from build123d import *

# Parameters (mm, degrees)
SKETCH1_R           = 5.5
BOSS_EXTRUDE1_DEPTH = 11
SKETCH3_R           = 15
BOSS_EXTRUDE2_DEPTH = 2
SKETCH4_R           = 15.011076053
SKETCH4_R_2         = 13.011076053
BOSS_EXTRUDE3_DEPTH = 59
SKETCH5_R           = 15.011076053
BOSS_EXTRUDE4_DEPTH = 2
CAVITY1_OUTLINE_R   = 1.25
CAVITY1_DEPTH       = 8
SKETCH6_R           = 1.25
CUT_EXTRUDE1_DEPTH  = 8


# Read off the part's stored shape, not the designer's step: Cavity1
with BuildPart() as part:
    # Sketch1 → Boss-Extrude1 (new body)
    with BuildSketch(Plane.XY):
        with Locations((0.700759494, -0.350379747)):
            Circle(SKETCH1_R)
    boss_extrude1 = extrude(amount=BOSS_EXTRUDE1_DEPTH)

    # Sketch3 → Boss-Extrude2 (add)
    with BuildSketch(Plane.XY.offset(11)):
        with Locations((0.700759494, -0.350379747)):
            Circle(SKETCH3_R)
    extrude(amount=BOSS_EXTRUDE2_DEPTH)

    # Sketch4 → Boss-Extrude3 (add)
    with BuildSketch(Plane.XY.offset(13)):
        with Locations((0.700759494, -0.350379747)):
            Circle(SKETCH4_R)
        with Locations((0.700759494, -0.350379747)):
            Circle(SKETCH4_R_2, mode=Mode.SUBTRACT)
    extrude(amount=BOSS_EXTRUDE3_DEPTH)

    # Sketch5 → Boss-Extrude4 (add)
    with BuildSketch(Plane.XY.offset(72)):
        with Locations((0.700759494, -0.350379747)):
            Circle(SKETCH5_R)
    extrude(amount=BOSS_EXTRUDE4_DEPTH)

    # Mirror1: Boss-Extrude1 across plane
    add(boss_extrude1.mirror(Plane.XY.offset(42.5)))

    # Cavity1 outline → Cavity1 (cut)
    with BuildSketch(Plane.XY):
        with BuildLine():
            Line((3.338761962, -0.602258645), (0.613426942, 2.29818081))
            ThreePointArc((0.613426942, 2.29818081), (-1.113870906, 1.580841761), (-1.937242974, -0.098500849))
            Line((-1.937242974, -0.098500849), (0.788092045, -2.998940304))
            ThreePointArc((0.788092045, -2.998940304), (2.515389893, -2.281601255), (3.338761962, -0.602258645))
        make_face()
        with Locations((0.700759494, -0.350379747)):
            Circle(CAVITY1_OUTLINE_R, mode=Mode.SUBTRACT)
    extrude(amount=CAVITY1_DEPTH, mode=Mode.SUBTRACT)

    # Sketch6 → Cut-Extrude1 (cut)
    with BuildSketch(Plane(origin=(0, 0, 0), x_dir=(-1, 0, 0), z_dir=(0, 0, -1))):
        with Locations((-0.700759494, -0.350379747)):
            Circle(SKETCH6_R)
    extrude(amount=-CUT_EXTRUDE1_DEPTH, mode=Mode.SUBTRACT)


solid = part.part
Design review of the part built by this model. Coordinates are the model's own, in mm. A direction names the side the tool comes from. Round coordinates to 2 decimals unless told otherwise and drop trailing zeros. Write each loop counter-clockwise with the first axis right and the second up, starting at its lowest first coordinate (ties: lowest second). Pieces come first, ordered by that corner, then holes.
Item 1: Consider section C-C on z = 6.5. Give the boundary of the cut face in (x, y), and give its area (3 significant figures).
Item 2: Draft analysis for pull direction Z (two halves, no side actions). For faces 5 (the flat face through (1, 0, 8)), 6 (the flat face through (1, 0, 13)), 7 (the cylindrical face through (-0.49, -5.72, 79.58)), state which applies: released by +Z, released by -Z, zero draft, split by the parting line, or undercut.
Item 3: For pin 1 Ø1 at (y, z) = (7, 26.5) entering from -X; pin 2 Ø5 at (y, z) = (6.5, 75.5) entering from -X; pin 3 Ø15 at (x, y) = (8, -1) entering from -Z; pin 4 Ø3 at (x, y) = (3, 10) entering from +Z, all flat-tipped, find the tip position at first contact; note any pin that passes through.
Item 4: For faces 1 (the flat face through (3, 0, 0)), 2 (the cylindrical face through (-0.49, -5.72, 5.42)), 3 (the flat face through (7, 0, 74)), 4 (the flat face through (1, 0, 72)), list the 3-axis set-ups (+Z, -Z, +X, -X, +Y, -Y) from which the entire face can be reached by the end or side of a thin tool; tool diameter is ignored.
Item 5: Wall thickness on L1, parallel to Z at x = -10, y = -2; L2, parallel to Z at x = -2.5, y = 3.5; L3, parallel to X at y = 0, z = 21: over which ranges is each line inside the solid? List them lowest first.
Check values:
1. outline: circle Ø11 at (0.7, -0.35); hole (-1.94, -0.1) - (0.79, -3) arc R2.65 ccw to (3.34, -0.6) - (0.61, 2.3) arc R2.65 ccw to start
1. area: 77.9 mm2
2. face 5: released by -Z
2. face 6: undercut
2. face 7: zero draft
3. pin 1: stops at x = -12.66
3. pin 2: stops at x = -13.51
3. pin 3: stops at z = 0
3. pin 4: stops at z = 74
4. face 1: -Z, +X, -X, +Y, -Y
4. face 2: -Z
4. face 3: +Z
4. face 4: none
5. L1: z = 11 to 13, 72 to 74
5. L2: z = 0 to 13, 72 to 85
5. L3: x = -14.31 to -12.31, 13.71 to 15.71
